Geometry: final body of the model. Coordinates: model frame, mm. Give positions to 0.01 mm unless a question says otherwise; leave off trailing zeros. Loops run counter-clockwise (first coordinate to the right, second up) from the corner with the lowest first, then second, coordinate; pieces in that order, holes last. Notation, with made-up numbers: (-0.5, 66) - (35.5, 66) arc R14 cw to (35.5, 78) - close; hole circle Ø1 at (55.5, -17). An arc over 180 degrees is marked (long way). Answer in a Markdown table with one row per item.
Autodesk Inventor part; units mm, degrees
ref_plane "YZ Plane" through (0, 0, 0) normal (1, 0, 0) x (0, 1, 0)
ref_plane "XZ Plane" through (0, 0, 0) normal (0, 1, 0) x (-1, 0, 0)
ref_plane "XY Plane" through (0, 0, 0) normal (0, 0, 1) x (1, 0, 0)
sketch "Sketch1" plane through (0, 0, 0) normal (0, 1, 0) x (-1, 0, 0)
  circle A0 centre (0, 0) radius 16.45
  circle A1 centre (0, 0) radius 8.55
  dimension "d0" = 32.9
  dimension "d1" = 17.1
extrude "Extrusion1" add sketch "Sketch1" along normal blind 2.5
sketch "Sketch2" plane through (0, 2.5, 0) normal (0, 1, 0) x (1, 0, 0)
  circle A0 centre (0, 0) radius 12.475
  line L0 (0, 0) -> (4.774, -11.5254)
  line L1 (0, 0) -> (21.8352, 0) construction
  line L2 (0, 0) -> (4.774, 11.5254)
  line L3 (0, 0) -> (76.5, 0) construction
  point P0 (-9.8971, -7.5943)
  point P1 (-9.8971, 7.5943)
  point P2 (4.774, 11.5254)
  dimension "d4" = 24.95
  dimension "d5" = 67.5
  dimension "d7" = 67.5
  dimension "d10" = 225
hole "Hole1" at (4.774, 2.5, 11.5254) at (-9.8971, 2.5, 7.5943) at (-9.8971, 2.5, -7.5943) at (4.774, 2.5, -11.5254) direction (0, -1, 0) diameter 3.2 depth 4 tip angle 118
chamfer "Chamfer1" distance 1.2 distance2 1 4 edges at (4.774, 2.5, -13.1254) (-9.8971, 2.5, -9.1943) (4.774, 2.5, 9.9254) (-9.8971, 2.5, 5.9943) measured on face at (-5.8151, 2.5, -10.6262)
properties part number "Simple_Mouting_Bracket"
Q1. Cut plane B-B (x = 0). Output: boundary loops of the cut face in (y, z).
Check values:
| item | result |
|---|---|
| outline | (0, -16.45) - (2.5, -16.45) - (2.5, -8.55) - (0, -8.55) - close; (0, 8.55) - (2.5, 8.55) - (2.5, 16.45) - (0, 16.45) - close |
Q2. Cut plane A-A (z = 0). Output: boundary loops of the cut face in (x, y), and give its area (3 significant figures).
Check values:
| item | result |
|---|---|
| outline | (-16.45, 0) - (-8.55, 0) - (-8.55, 2.5) - (-16.45, 2.5) - close; (8.55, 0) - (16.45, 0) - (16.45, 2.5) - (8.55, 2.5) - close |
| area | 39.5 mm² |
Q3. Cut plane C-C (y = 0.8). Output: boundary loops of the cut face in (x, z), and give its area (3 significant figures).
Check values:
| item | result |
|---|---|
| outline | circle Ø32.9 at (0, 0); hole circle Ø3.2 at (-9.9, -7.59); hole circle Ø3.2 at (-9.9, 7.59); hole circle Ø17.1 at (0, 0); hole circle Ø3.2 at (4.77, -11.53); hole circle Ø3.2 at (4.77, 11.53) |
| area | 588 mm² |
Q4. Material intervals for line 1 along X through (y, z) = (1.2, -7); line 2 along Z through (x, y) = (-11.5, 2.1); line 3 along Z through (x, y) = (-9, 1.8), sorted ascending.
Check values:
| item | result |
|---|---|
| line 1 | -14.89 to -11.38, -8.41 to -4.91, 4.91 to 14.89 |
| line 2 | -11.76 to -9.27, -5.92 to 5.92, 9.27 to 11.76 |
| line 3 | -13.77 to -9.34, -5.85 to 5.85, 9.34 to 13.77 |
Q5. First-contact query: pin 1 (1.5 mm diameter, centred on y = 0.5, z = -2, fed in from +X); pin 2 (5 mm diameter, centred on x = 4.77, z = -11.53, fed in from +Y); pin 3 (1.5 mm diameter, centred on y = 0.5, z = -2, fed in from -X). Flat tips, straight axial feed; report the tip coordinate or a pass-through.
Check values:
| item | result |
|---|---|
| pin 1 | x = 16.4 |
| pin 2 | y = 2.26 |
| pin 3 | x = -16.4 |
Q6. Draft query along Z for faces 1 (the flat face through (-7, 0, -7)), 2 (the cylindrical face through (3.566, 1.232, 16.059)), 3 (the cylindrical face through (-8.155, 1.232, -2.568)). Return one class per face: pulls with the +Z half, pulls with the -Z half, needs draft (parallel to the pull), parting line crosses it, or undercut.
Check values:
| item | result |
|---|---|
| face 1 | needs draft |
| face 2 | parting line crosses it |
| face 3 | undercut |
Q7. Cut plane D-D (z = -8). Give the number of separate pieces and of enclosed holes in the cut face, and give its area (3 significant figures).
Check values:
| item | result |
|---|---|
| separate pieces | 3 |
| enclosed holes | 0 |
| area | 47.8 mm² |
